Source: three-view drawing plus pictorial views. Frame: mm from the lowest corner of the part. A direction names the side the tool comes from. Round coordinates to 2 decimals unless told otherwise and drop trailing zeros. Order: outer loops, then holes, each group sorted by start corner. A loop starts at its lowest first (then second) coordinate and runs counter-clockwise, first axis right, second up. Notation, with made-up numbers: (15, 5.5) -> (58, 5.5) arc R9 ccw to (58, 21.5) -> close; hole circle Ø2 at (-1, -10.5). An arc over 180 degrees is marked (long way). Use a Markdown table: item, result.
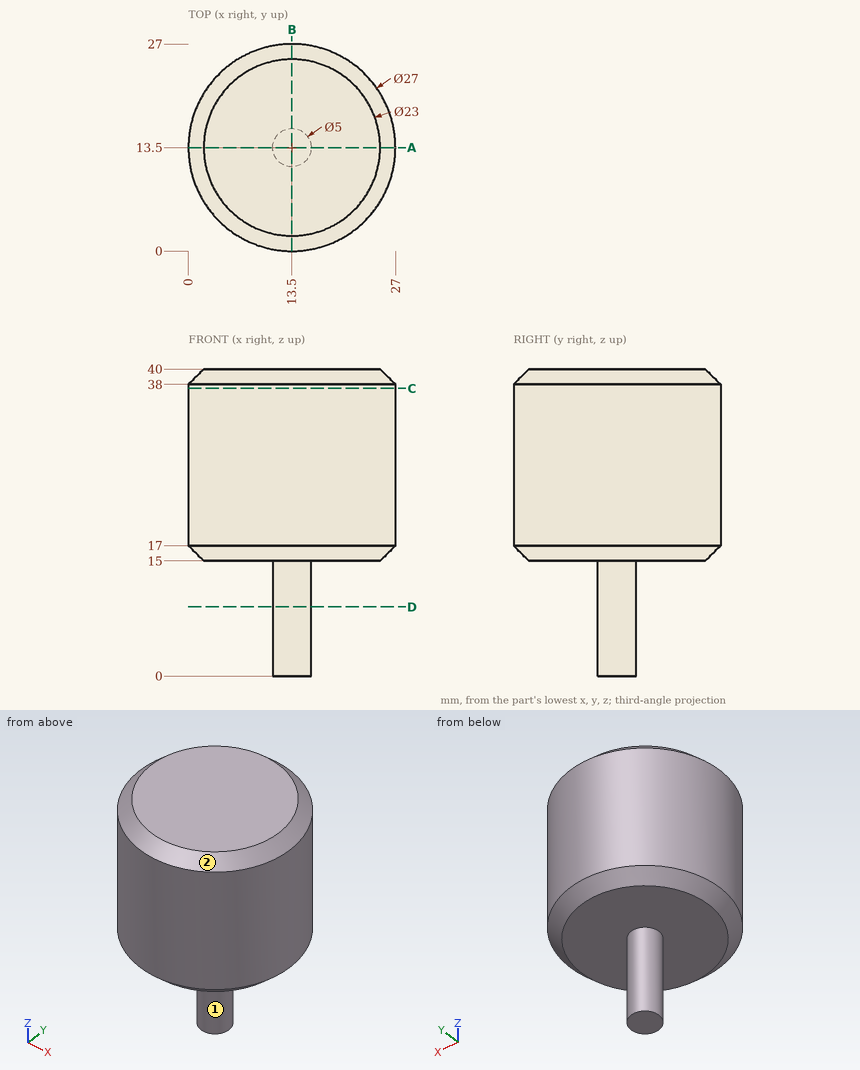
1) Cut plane C-C on z = 37.5. Return loops of the section in (x, y).
Results found:
| item | result |
|---|---|
| outline | circle Ø27 at (13.5, 13.5) |
2) Pin query (flat end, axial travel): pin 1 Ø1 at (y, z) = (6, 35) entering from -X; pin 2 Ø1.5 at (x, z) = (15, 23.5) entering from +Y; pin 3 Ø3 at (y, z) = (3, 32) entering from +X. Return the tip coordinate at first contact, or that it passes through.
Results found:
| item | result |
|---|---|
| pin 1 | stops at x = 1.96 |
| pin 2 | stops at y = 26.98 |
| pin 3 | stops at x = 23.56 |
3) Set-up query: the marked faces 1 and 2. Return all of +Z, -Z, +X, -X, +Y, -Y with unobstructed straight access to the full face (end or side cutting, diameter ignored); none if empty.
Results found:
| item | result |
|---|---|
| face 1 | -Z |
| face 2 | +Z |
4) Line query: L1, parallel to Z at x = 22, y = 16; L2, parallel to X at y = 14, z = 34; L3, parallel to Z at x = 25.25, y = 13.5. Output: solid intervals per line, ascending. Write a range as [from, to].
Results found:
| item | result |
|---|---|
| L1 | z = [15, 40] |
| L2 | x = [0.01, 26.99] |
| L3 | z = [15.25, 39.75] |
5) Cut plane A-A on y = 13.5. Return loops of the section in (x, z), and give its area (3 significant figures).
Results found:
| item | result |
|---|---|
| outline | (0, 17) -> (2, 15) -> (11, 15) -> (11, 0) -> (16, 0) -> (16, 15) -> (25, 15) -> (27, 17) -> (27, 38) -> (25, 40) -> (2, 40) -> (0, 38) -> close |
| area | 742 mm² |
6) Cut plane D-D on z = 9. Return loops of the section in (x, y).
Results found:
| item | result |
|---|---|
| outline | circle Ø5 at (13.5, 13.5) |
